Job drawing, mm, ordinate dimensions from the low corner. One solid piece. A direction names the side the tool comes from. Give positions to 0.01 mm unless a question says otherwise; leave off trailing zeros. Write each loop counter-clockwise with the first axis right and the second up, starting at its lowest first coordinate (ties: lowest second). Pieces come first, ordered by that corner, then holes. Notation, with made-up numbers: (9, 15) - (26, 15) arc R7 cw to (26, 26) - close; hole circle Ø2 at (7, -26.75). An arc over 180 degrees is marked (long way). Answer in a Markdown table with one row per item. Add a question column.
1. Probe line 1 along Z through (x, y) = (9, 29); line 2 along Y through (x, z) = (22.25, 30.5); line 3 along Y through (x, z) = (16, 2.5). List the from-to ranges inside material, lowest first.
2. Band-saw the part on C-C on x = 12. Write the cut outline in (y, z), plus the area to 3 significant figures.
3. Band-saw the part on A-A on z = 30.5. Write the cut outline in (x, y).
4. Pull direction Z, two halves, no side cores. Call the marked faces 1, 2, 3 and 4: released by +Z, released by -Z, zero draft, split by the parting line, or undercut.
5. Drop flat-ended pins along their axis: pin 1 Ø4.5 at (y, z) = (3, 23.5) entering from -X; pin 2 Ø1.5 at (x, y) = (16, 27.25) entering from -Z; pin 3 Ø5 at (x, z) = (5, 26.5) entering from -Y; pin 4 Ø1 at (x, z) = (5, 10.5) entering from +Y. Give the stop position or say it passes through.
6. Band-saw the part on B-B on y = 4. Write the cut outline in (x, z).
7. Band-saw the part on D-D on x = 4.75. Write the cut outline in (y, z).
8. Which spindle directions (+Z, -Z, +X, -X, +Y, -Y) get a long thin tool onto all of the face, cutting with end or side? Do the marked faces 5, 6, 7, 8 and 9. Say none if no direction does.
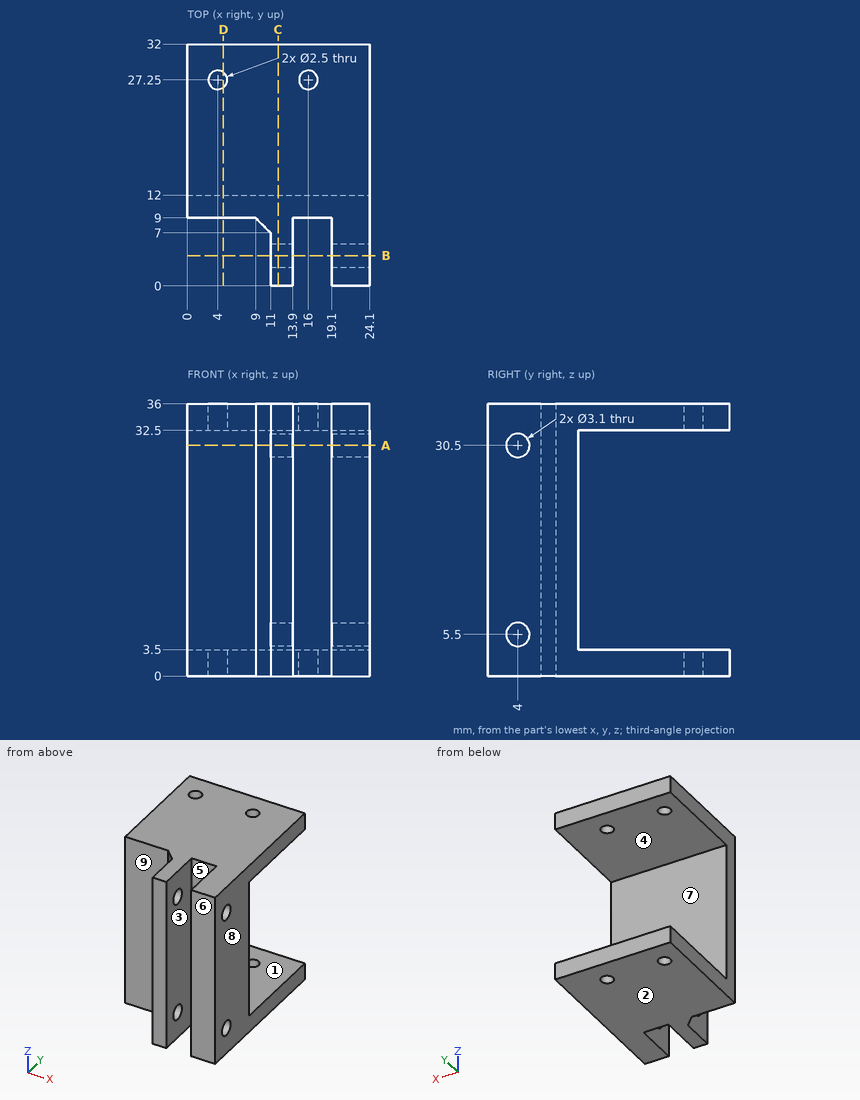
Values:
| question | item | result |
|---|---|---|
| 1 | line 1 | z = 0 to 3.5, 32.5 to 36 |
| 1 | line 2 | y = 0 to 2.45, 5.55 to 12 |
| 1 | line 3 | y = 9 to 26, 28.5 to 32 |
| 2 | outline | (0, 0) - (32, 0) - (32, 3.5) - (12, 3.5) - (12, 32.5) - (32, 32.5) - (32, 36) - (0, 36) - close; hole circle Ø3.1 at (4, 5.5); hole circle Ø3.1 at (4, 30.5) |
| 2 | area | 557 mm² |
| 3 | outline | (0, 9) - (9, 9) - (11, 7) - (11, 5.55) - (13.9, 5.55) - (13.9, 9) - (19.1, 9) - (19.1, 5.55) - (24.1, 5.55) - (24.1, 12) - (0, 12) - close; (11, 0) - (13.9, 0) - (13.9, 2.45) - (11, 2.45) - close; (19.1, 0) - (24.1, 0) - (24.1, 2.45) - (19.1, 2.45) - close |
| 4 | face 1 | undercut |
| 4 | face 2 | released by -Z |
| 4 | face 3 | zero draft |
| 4 | face 4 | undercut |
| 5 | pin 1 | stops at x = 11 |
| 5 | pin 2 | passes through |
| 5 | pin 3 | stops at y = 9 |
| 5 | pin 4 | stops at y = 12 |
| 6 | outline | (11, 0) - (13.9, 0) - (13.9, 3.95) - (11, 3.95) - close; (11, 7.05) - (13.9, 7.05) - (13.9, 28.95) - (11, 28.95) - close; (11, 32.05) - (13.9, 32.05) - (13.9, 36) - (11, 36) - close; (19.1, 0) - (24.1, 0) - (24.1, 3.95) - (19.1, 3.95) - close; (19.1, 7.05) - (24.1, 7.05) - (24.1, 28.95) - (19.1, 28.95) - close; (19.1, 32.05) - (24.1, 32.05) - (24.1, 36) - (19.1, 36) - close |
| 7 | outline | (9, 0) - (26.25, 0) - (26.25, 3.5) - (12, 3.5) - (12, 32.5) - (26.25, 32.5) - (26.25, 36) - (9, 36) - close; (28.25, 0) - (32, 0) - (32, 3.5) - (28.25, 3.5) - close; (28.25, 32.5) - (32, 32.5) - (32, 36) - (28.25, 36) - close |
| 8 | face 5 | +Z, -Z, -Y |
| 8 | face 6 | +Z, -Z, +X, -X, -Y |
| 8 | face 7 | +X, -X, +Y |
| 8 | face 8 | +Z, -Z, +X, +Y, -Y |
| 8 | face 9 | +Z, -Z, -X, -Y |
